Could you check a few things on this model? Use its own coordinates, in mm. A direction names the side the tool comes from. Give positions to 0.01 mm unless a question says otherwise; leave off trailing zeros. Loops run counter-clockwise (first coordinate to the right, second up) from the corner with the lowest first, then second, coordinate; pieces in that order, holes last. Notation, with made-up numbers: (59.25, -24) - (109.25, -24) arc R27 cw to (109.25, 4) - close; hole circle Ø5 at (-11, 15.25). An arc over 180 degrees is marked (long way). Use CSV: the item, a comma, the result in double quotes.
Autodesk Inventor part; units mm, degrees
ref_plane "Work Plane1" through (0, 3.175, 15) normal (0, 1, 0) x (1, 0, 0)
ref_plane "Work Plane3" through (11.5, -12, 0) normal (1, 0, 0) x (0, 0, -1)
ref_plane "YZ Plane" through (0, 0, 0) normal (1, 0, 0) x (0, 1, 0)
sketch "Sketch1" plane through (0, 0, 0) normal (0, 0, 1) x (1, 0, 0)
  line L0 (-4.3, 0) -> (27.3, 0)
  line L1 (27.5, -0.2) -> (27.5, -5.5)
  line L2 (-4.3, -12) -> (27.3, -12)
  line L3 (27.5, -6.5) -> (27.5, -11.8)
  line L4 (-4.5, -0.2) -> (-4.5, -5.5)
  line L5 (-4.5, -6.5) -> (-4.5, -11.8)
  line L6 (-4.5, 0) -> (-1.071, 0)
  line L7 (-1.071, 0) -> (-1.071, -12)
  line L8 (-1.071, -12) -> (-4.5, -12)
  line L9 (-4.5, -12) -> (-4.5, 0)
  arc A0 (-3.366, -6.5) -> (-3.366, -5.5) centre (-2.5, -6) ccw
  circle A1 centre (-2.5, -6) radius 1
  line L10 (27.5, -12) -> (24.071, -12)
  line L11 (24.071, -12) -> (24.071, 0)
  line L12 (24.071, 0) -> (27.5, 0)
  line L13 (27.5, 0) -> (27.5, -12)
  arc A2 (26.366, -5.5) -> (26.366, -6.5) centre (25.5, -6) ccw
  circle A3 centre (25.5, -6) radius 1
  line L14 (-1.071, 0) -> (-4.5, 0)
  line L15 (-4.5, 0) -> (-4.5, 1.905)
  line L16 (-4.5, 1.905) -> (-1.071, 1.905)
  line L17 (-1.071, 1.905) -> (-1.071, 0)
  line L18 (11.5, 0) -> (11.5, -12) construction
  line L19 (27.5, 0) -> (24.071, 0)
  line L20 (24.071, 0) -> (27.5, 0)
  line L21 (27.5, 0) -> (27.5, 1.905)
  line L22 (27.5, 1.905) -> (24.071, 1.905)
  line L23 (24.071, 1.905) -> (24.071, 0)
  line L24 (-4.5, 1.905) -> (-1.071, 1.905)
  line L25 (-1.071, 1.905) -> (-1.071, 5.08)
  line L26 (-1.071, 5.08) -> (-4.5, 5.08)
  line L27 (-4.5, 5.08) -> (-4.5, 1.905)
  line L28 (24.071, 1.905) -> (27.5, 1.905)
  line L29 (27.5, 1.905) -> (27.5, 5.08)
  line L30 (27.5, 5.08) -> (24.071, 5.08)
  line L31 (24.071, 5.08) -> (24.071, 1.905)
  point P0 (0, 0)
  dimension "d0" = 3.429
  dimension "d1" = 3.429
  dimension "d2" = 1.905
  dimension "d8" = 3.175
  dimension "d9" = 3.175
extrude "Extrusion1" add sketch "Sketch1" along normal blind 1.905 contours L6 L15 L16 L17 L0 | L0 L7 L2 L8 L9 L5 L4 L6 | L23 L22 L21 L12 L0 | L0 L12 L13 L1 L3 L10 L2 L11 | L16 L27 L26 L25 | L31 L30 L29 L22
ref_plane "Work Plane1" through (0, 3.175, 15) normal (0, 1, 0) x (1, 0, 0)
sketch "Sketch2" plane through (0, 3.175, 15) normal (0, 1, 0) x (1, 0, 0)
  line L0 (-1.071, 15) -> (-4.5, 15)
  line L1 (-4.5, 15) -> (-4.5, 13.095)
  line L2 (-1.071, 13.095) -> (-4.5, 13.095)
  line L3 (-1.071, 15) -> (-1.071, 13.095)
  line L4 (27.5, 15) -> (24.071, 15)
  line L5 (24.071, 15) -> (24.071, 13.095)
  line L6 (27.5, 13.095) -> (24.071, 13.095)
  line L7 (27.5, 15) -> (27.5, 13.095)
  line L8 (22.8, 0) -> (0.2, 0)
  line L9 (-4.5, 13.095) -> (27.5, 13.095)
  line L10 (27.5, -3.175) -> (-4.5, -3.175)
  line L11 (-4.5, 11.19) -> (-1.071, 11.19)
  line L12 (-1.071, 11.19) -> (-1.071, 0)
  line L13 (-1.071, 0) -> (-4.5, 0)
  line L14 (27.5, 0) -> (24.071, 0)
  line L15 (24.071, 0) -> (24.071, 11.19)
  line L16 (24.071, 11.19) -> (27.5, 11.19)
  line L17 (23, 15) -> (23, 5)
  line L18 (0, 5) -> (0, 15)
  line L19 (-1.071, 15) -> (-1.071, 13.095)
  line L20 (24.071, 15) -> (24.071, 13.095)
  arc A0 (-1.071, 7.761) -> (-4.5, 11.19) centre (-4.5, 7.761) ccw
  arc A1 (-4.5, 0) -> (-1.071, 3.429) centre (-4.5, 3.429) ccw
  arc A2 (27.5, 11.19) -> (24.071, 7.761) centre (27.5, 7.761) ccw
  arc A3 (24.071, 3.429) -> (27.5, 0) centre (27.5, 3.429) ccw
  line L21 (-4.5, -3.175) -> (-4.5, 0)
  line L22 (-4.5, 11.19) -> (-4.5, 13.095)
  line L23 (27.5, 13.095) -> (27.5, 11.19)
  line L24 (27.5, 0) -> (27.5, -3.175)
  dimension "d5" = 3.175
  dimension "d13" = 1.905
extrude "Extrusion2" add sketch "Sketch2" along normal blind 1.905 contours L9 L6 L23 L16 L15 L14 L24 L10 L21 L13 L12 L11 L22 L2 | L11 L12 A0 | L12 L13 A1 | A2 L15 L16 | A3 L14 L15
sketch "Sketch6" plane through (0, 3.175, 15) normal (0, -1, 0) x (1, 0, 0)
  line L0 (0.2, 0) -> (22.8, 0)
  line L1 (-4.5, -15) -> (-4.5, 3.175)
  line L2 (27.5, 3.175) -> (-4.5, 3.175)
  line L3 (-4.5, 3.175) -> (-4.5, 1.27)
  line L4 (-4.5, 1.27) -> (27.5, 1.27)
  line L5 (27.5, 1.27) -> (27.5, 3.175)
  line L6 (27.5, 3.175) -> (27.5, -13.095)
  line L7 (-4.5, 3.175) -> (27.5, 3.175)
  point P0 (0, -15)
  dimension "d10" = 1.905
extrude "Extrusion3" add sketch "Sketch6" along normal up to surface (15.175 mm away)
fillet "Fillet1" radius 3.175 4 edges at (-4.5, 4.1275, 3.81) (-4.5, 4.1275, 15) (27.5, 4.1275, 15) (27.5, 4.1275, 3.81)
sketch "Sketch7" plane through (-4.5, 5.08, 18.175) normal (0, 0, 1) x (1, 0, 0)
  line L0 (32, -17.08) -> (32, 0)
  line L1 (0, 0) -> (32, 0)
  line L2 (0, -17.08) -> (0, 0)
  line L3 (0, -17.08) -> (32, -17.08)
  line L4 (31.8064, -17.08) -> (0.1936, -17.08) construction
  line L5 (32, -17.08) -> (32, 0) construction
  circle A0 centre (10.5, -11.08) radius 1.5875
  circle A1 centre (10.5, -11.08) radius 3.75
  point P0 (4.5, -5.08)
  dimension "d15" = 3.175
sketch "Sketch8" plane through (24.071, 5.08, 0) normal (0, 1, 0) x (1, 0, 0)
  arc A0 (1.7804, -4.2323) -> (3.429, -1.4483) centre (0.254, -1.4483) ccw
  line L0 (3.429, 0) -> (3.429, -1.4483)
  line L1 (3.429, 0) -> (0, 0)
  line L2 (0, 0) -> (0, -1.905)
  line L3 (0, -1.905) -> (-25.142, -1.905)
  line L4 (-25.142, 0) -> (-25.142, -1.905)
  line L5 (-25.142, 0) -> (-28.571, 0)
  line L6 (-28.571, 0) -> (-28.571, -1.4483)
  arc A1 (-28.571, -1.4483) -> (-26.9224, -4.2323) centre (-25.396, -1.4483) ccw
  arc A2 (-25.142, -7.239) -> (-26.9224, -4.2323) centre (-28.571, -7.239) ccw
  line L7 (-25.142, -7.239) -> (-25.142, -11.571)
  arc A3 (-26.9224, -14.5777) -> (-25.142, -11.571) centre (-28.571, -11.571) ccw
  arc A4 (-26.9224, -14.5777) -> (-28.571, -17.3617) centre (-25.396, -17.3617) ccw
  line L8 (-28.571, -17.3617) -> (-28.571, -18.175)
  line L9 (-28.571, -18.175) -> (3.429, -18.175)
  line L10 (3.429, -18.175) -> (3.429, -17.3617)
  arc A5 (3.429, -17.3617) -> (1.7804, -14.5777) centre (0.254, -17.3617) ccw
  arc A6 (0, -11.571) -> (1.7804, -14.5777) centre (3.429, -11.571) ccw
  line L11 (0, -11.571) -> (0, -7.239)
  arc A7 (1.7804, -4.2323) -> (0, -7.239) centre (3.429, -7.239) ccw
  line L12 (-25.142, -7.239) -> (-25.142, -11.571) construction
  circle A8 centre (-18.071, -9.405) radius 1.5875
  line L13 (-21.821, 16.1332) -> (-14.321, 16.1332)
  line L14 (-18.071, 16.1332) -> (-18.071, -9.3987) construction
  line L15 (-25.142, -9.405) -> (0, -9.405) construction
  point P0 (-24.071, 0)
  dimension "d16" = 3.175
extrude "Extrusion4" cut sketch "Sketch8" against normal up to next contours A8
extrude "Extrusion5" cut sketch "Sketch7" against normal up to next contours A0
ref_plane "Work Plane3" through (11.5, -12, 0) normal (1, 0, 0) x (0, 0, -1)
mirror "Mirror1" about plane through (11.5, -12, 0) normal (1, 0, 0) of "Extrusion5"
mirror "Mirror2" about plane through (11.5, -12, 0) normal (1, 0, 0) of "Extrusion4"
properties part number "Servo_vice"
1) Suppose I cut it at A-A (x = 6). Please give me the cut outline in (y, z) (1 decimal).
Answer below:
outline,"(-12, 16.3) - (-7.6, 16.3) - (-7.6, 18.2) - (-12, 18.2) - close; (-4.4, 16.3) - (3.2, 16.3) - (3.2, 11) - (5.1, 11) - (5.1, 18.2) - (-4.4, 18.2) - close; (3.2, 1.9) - (5.1, 1.9) - (5.1, 7.8) - (3.2, 7.8) - close"
2) Suppose I cut it at B-B (y = -2.25). Please give me the cut outline in (x, z) (3 decimals), plus the area to 3 significant figures.
Answer below:
outline,"(-4.5, 0) - (-1.071, 0) - (-1.071, 1.905) - (-4.467, 1.905) arc R3.175 ccw to (-4.5, 1.448) - close; (-4.5, 17.362) arc R3.175 ccw to (-4.306, 16.27) - (27.306, 16.27) arc R3.175 ccw to (27.5, 17.362) - (27.5, 18.175) - (-4.5, 18.175) - close; (24.071, 0) - (27.5, 0) - (27.5, 1.448) arc R3.175 ccw to (27.467, 1.905) - (24.071, 1.905) - close"
area,"73.9 mm2"
3) Suppose I cut it at C-C (z = 1). Please give me the cut outline in (x, y), plus the area to 3 significant figures.
Answer below:
outline,"(-4.5, -12) - (-1.07, -12) - (-1.07, 5.08) - (-4.5, 5.08) - close; (24.07, -12) - (27.5, -12) - (27.5, 5.08) - (24.07, 5.08) - close; hole (-3.37, -6.5) arc R1 ccw (long way) to (-3.37, -5.5) arc R1 ccw to start; hole circle Ø2 at (25.5, -6)"
area,"111 mm2"
4) I need wall thicknesses on line 1 along X through (y, z) = (-6, 0.9); line 2 along Z through (x, y) = (26, 1) (3 decimals); line 3 along Y through (x, z) = (-2.5, 1.45). Which ranges of each line are inside material? Lowest first, please.
Answer below:
line 1,"x = -4.5 to -3.5, -1.5 to -1.07, 24.07 to 24.5, 26.5 to 27.5"
line 2,"z = 0 to 1.905, 16.27 to 18.175"
line 3,"y = -12 to -7, -5 to 5.08"
5) Suppose I cut it at D-D (x = 21). Please give me the cut outline in (y, z) (3 decimals), plus the area to 3 significant figures.
Answer below:
outline,"(-12, 16.27) - (3.175, 16.27) - (3.175, 1.905) - (5.08, 1.905) - (5.08, 18.175) - (-12, 18.175) - close"
area,"59.9 mm2"
6) Which directions (+Z, -Z, +X, -X, +Y, -Y) give clear straight access to the entire face, cutting with the end or side of a thin tool? Please do faces 5 (the cylindrical face through (27.494, -0.89, 1.645)), 6 (the cylindrical face through (-4.485, -0.89, 1.754)), 7 (the flat face through (-3, -4, 1.905)), 8 (the cylindrical face through (-1.5, -6, 0.9)).
Answer below:
face 5,"+X, +Y, -Y"
face 6,"-X, +Y, -Y"
face 7,"+X, -X, -Y"
face 8,"-Z"
7) I'm going to push flat-ended pins straight in: P1, Ø4, axis at x = 6, z = 9.405, coming from the +Y side; P2, Ø1.5, axis at y = 4, z = 9, coming from the +X side; P3, Ø4, axis at x = 17, z = 9.405, coming from the -Y side (3 decimals); P4, Ø1.6, axis at x = 25.5, y = -6, coming from the -Z side. Where does each tip first touch, or does it pass through?
Answer below:
P1,"stops at y = 5.08"
P2,"stops at x = 24.07"
P3,"stops at y = 3.175"
P4,"stops at z = 16.27"
8) We'd pull the mould along X, two halves only. Please class faces 1 (the flat face through (26, -3, 0)), 2 (the cylindrical face through (-1.54, 4.11, 13.3)), 3 (the cylindrical face through (-3.5, -6, 0.9)), 4 (the cylindrical face through (16.267, 4.141, 7.997)): +X half, -X half, draft (parallel to the pull), parting line (faces both ways), or undercut.
Answer below:
face 1,"draft"
face 2,"-X half"
face 3,"undercut"
face 4,"undercut"
